Geometry check sheet. Reference: the model listing, model coordinates, mm. A direction names the side the tool comes from. Give positions to 0.01 mm unless a question says otherwise; leave off trailing zeros. Write each loop counter-clockwise with the first axis right and the second up, starting at its lowest first coordinate (ties: lowest second). Pieces come first, ordered by that corner, then holes. Notation, with made-up numbers: M -15,1 L 41,1 A32 cw 41,30 Z; hole C -8,-9 d5. An arc over 180 degrees is marked long. Write each question's results on one line, items separated by ' | '.
```python
from build123d import *

# Parameters (mm, degrees)
ESBO_O1_W       = 24.65
ESBO_O1_H       = 16
ESBO_O2_W       = 30
ESBO_O2_H       = 12
EXTRUS_O1_DEPTH = 25.1
CHANFRO1_SIZE   = 3
EXTRUS_O2_DEPTH = 1
ESBO_O5_W       = 8.5
ESBO_O5_H       = 6
EXTRUS_O3_DEPTH = 0.3
ESBO_O6_W       = 6.5
ESBO_O6_H       = 1
EXTRUS_O4_DEPTH = 10
ESBO_O7_R       = 2
EXTRUS_O5_DEPTH = 1
FILETE1_R       = 3
ESBO_O8_R       = 6
EXTRUS_O6_DEPTH = 2
ESBO_O9_R       = 3.5
EXTRUS_O7_DEPTH = 9.4
ESBO_O10_W      = 6.32455532
ESBO_O10_H      = 3.599019514
EXTRUS_O8_DEPTH = 6
ESBO_O11_W      = 30
ESBO_O11_H      = 9.10840564
EXTRUS_O9_DEPTH = 0.5
FILETE2_R       = 2


with BuildPart() as part:
    # Esboço1 → Revolução1 (revolve)
    with BuildSketch(Plane.XY, mode=Mode.PRIVATE) as revolu_o1_sk:
        with Locations((-12.325, 8)):
            Rectangle(ESBO_O1_W, ESBO_O1_H)
    revolve(revolu_o1_sk.sketch.rotate(Axis((0, 0, 0), (0, 1, 0)), 270), axis=Axis((0, 0, 0), (0, 1, 0)))

    # Esboço2 → Extrusão1 (add)
    with BuildSketch(Plane.XY):
        with Locations((0, 10)):
            Rectangle(ESBO_O2_W, ESBO_O2_H)
    extrude(amount=EXTRUS_O1_DEPTH)

    # Chanfro1
    chanfro1_edges = [part.edges().sort_by_distance(p)[0] for p in [
        (-15, 10, 25.1),
        (15, 10, 25.1),
    ]]
    chamfer(chanfro1_edges, length=CHANFRO1_SIZE)

    # Esboço4 → Extrusão2 (add)
    with BuildSketch(Plane.XY.offset(25.1)):
        Polygon((-12, 5), (-0.5, 5), (-0.5, 16), (0.5, 16), (0.5, 5), (12, 5), (12, 4), (-12, 4), align=None)
    extrude(amount=EXTRUS_O2_DEPTH)

    # Esboço5 → Extrusão3 (add)
    with BuildSketch(Plane.XY.offset(25.1)):
        with Locations((-7.75, 8)):
            Rectangle(ESBO_O5_W, ESBO_O5_H)
        with Locations((7.75, 8)):
            Rectangle(ESBO_O5_W, ESBO_O5_H)
    extrude(amount=EXTRUS_O3_DEPTH)

    # Esboço6 → Extrusão4 (add)
    with BuildSketch(Plane.XY.offset(25.4)):
        with Locations((-7.75, 8.5)):
            Rectangle(ESBO_O6_W, ESBO_O6_H)
        with Locations((7.75, 8.5)):
            Rectangle(ESBO_O6_W, ESBO_O6_H)
    extrude(amount=EXTRUS_O4_DEPTH)

    # Esboço7 → Extrusão5 (add)
    # profile 1 of 2: a face of its own
    with BuildSketch(Plane(origin=(0, 16, 0), x_dir=(1, 0, 0), z_dir=(0, 1, 0))):
        with BuildLine():
            ThreePointArc((-19.930990459, -14.504417235), (-23.303909287, -8.034320875), (-24.634983886, -0.860272594))
            Line((-24.634983886, -0.860272594), (-32, -1.117464624))
            Line((-32, -1.117464624), (-29.875626197, -14.851691567))
            Line((-29.875626197, -14.851691567), (-19.930990459, -14.504417235))
        make_face()
        with Locations(Location((-27.5, -11.35, 0), (0, 0, 270))):
            Circle(ESBO_O7_R, mode=Mode.SUBTRACT)
        with Locations(Location((-28.5, -4.35, 0), (0, 0, 270))):
            Circle(ESBO_O7_R, mode=Mode.SUBTRACT)
    # profile 2 of 2: a face of its own
    with BuildSketch(Plane(origin=(0, 16, 0), x_dir=(1, 0, 0), z_dir=(0, 1, 0))):
        with BuildLine():
            Line((32, -1.117464624), (24.634983886, -0.860272594))
            ThreePointArc((24.634983886, -0.860272594), (23.303909287, -8.034320875), (19.930990459, -14.504417235))
            Line((19.930990459, -14.504417235), (29.875626197, -14.851691567))
            Line((29.875626197, -14.851691567), (32, -1.117464624))
        make_face()
        with Locations(Location((27.5, -11.35, 0), (0, 0, 270))):
            Circle(ESBO_O7_R, mode=Mode.SUBTRACT)
        with Locations(Location((28.5, -4.35, 0), (0, 0, 270))):
            Circle(ESBO_O7_R, mode=Mode.SUBTRACT)
    extrude(amount=-EXTRUS_O5_DEPTH)

    # Filete1
    filete1_edges = [part.edges().sort_by_distance(p)[0] for p in [
        (-32, 15.5, 1.117464624),
        (-29.875626197, 15.5, 14.851691567),
        (32, 15.5, 1.117464624),
        (29.875626197, 15.5, 14.851691567),
    ]]
    fillet(filete1_edges, radius=FILETE1_R)

    # Esboço8 → Extrusão6 (add)
    with BuildSketch(Plane(origin=(0, 16, 0), x_dir=(1, 0, 0), z_dir=(0, 1, 0))):
        with Locations(Location((0, 12.65, 0), (0, 0, 90))):
            Circle(ESBO_O8_R)
    extrude(amount=EXTRUS_O6_DEPTH)

    # Esboço9 → Extrusão7 (add)
    with BuildSketch(Plane(origin=(0, 18, 0), x_dir=(1, 0, 0), z_dir=(0, 1, 0))):
        with Locations(Location((0, 12.65, 0), (0, 0, 270))):
            Circle(ESBO_O9_R)
    extrude(amount=EXTRUS_O7_DEPTH)

    # Esboço10 → Extrusão8 (cut)
    with BuildSketch(Plane(origin=(0, 27.4, 0), x_dir=(1, 0, 0), z_dir=(0, 1, 0))):
        with Locations((0, 9.350490243)):
            Rectangle(ESBO_O10_W, ESBO_O10_H)
    extrude(amount=-EXTRUS_O8_DEPTH, mode=Mode.SUBTRACT)

    # Esboço11 → Extrusão9 (cut)
    with BuildSketch(Plane(origin=(0, 16, 0), x_dir=(1, 0, 0), z_dir=(0, 1, 0))):
        with Locations((0, -24.114941559)):
            Rectangle(ESBO_O11_W, ESBO_O11_H)
    extrude(amount=-EXTRUS_O9_DEPTH, mode=Mode.SUBTRACT)

    # Filete2
    filete2_edges = [part.edges().sort_by_distance(p)[0] for p in [
        (4.5, 8.5, 35.4),
        (11, 8.5, 35.4),
        (-11, 8.5, 35.4),
        (-4.5, 8.5, 35.4),
    ]]
    fillet(filete2_edges, radius=FILETE2_R)


solid = part.part
```
Q1. Section check C-C (z = 0). Enter the section's corners in (x, y).
Answer key:
outline: M -24.65,0 L 24.65,0 L 24.65,16 L -24.65,16 Z
Q2. Material ranges on probe 1 along X at (y, z) = (15.3, 4.35); probe 2 along X at (y, z) = (8.5, 30); probe 3 along X at (y, z) = (15.8, 11.35), recorded low to high. Write a range as [from, to].
Answer key:
probe 1: x = [-31.5, -30.5], [-26.5, 26.5], [30.5, 31.5] | probe 2: x = [-11, -4.5], [4.5, 11] | probe 3: x = [-30.42, -29.5], [-25.5, 25.5], [29.5, 30.42]
Q3. Section check B-B (y = 13.25). Enter the section's corners in (x, z).
Answer key:
outline: M -15,19.56 A24.65 ccw long 15,19.56 L 15,22.1 L 12,25.1 L 0.5,25.1 L 0.5,26.1 L -0.5,26.1 L -0.5,25.1 L -12,25.1 L -15,22.1 Z
Q4. Depth check by flat-ended pin: P1, Ø1, axis at x = 0.5, z = -10.5, coming from the +Y side; P2, Ø3, axis at y = 6.5, z = -1, coming from the +X side; P3, Ø3.5, axis at x = 3, z = -11, coming from the +Y side; P4, Ø9.5, axis at x = 28.5, z = 9.5, coming from the -Y side. Enter the tip coordinate at first touch or a pass-through.
Answer key:
P1: stops at y = 21.4 | P2: stops at x = 24.65 | P3: stops at y = 27.4 | P4: stops at y = 15
Q5. Section check D-D (y = 10). Enter the section's corners in (x, z), then the cut area to 3 significant figures.
Answer key:
outline: M -15,19.56 A24.65 ccw long 15,19.56 L 15,22.1 L 12,25.1 L 12,25.4 L 3.5,25.4 L 3.5,25.1 L 0.5,25.1 L 0.5,26.1 L -0.5,26.1 L -0.5,25.1 L -3.5,25.1 L -3.5,25.4 L -12,25.4 L -12,25.1 L -15,22.1 Z | area: 1,970 mm2
Q6. Section check A-A (z = 27). Enter the section's corners in (x, y).
Answer key:
outline: M -11,8 L -4.5,8 L -4.5,9 L -11,9 Z; M 4.5,8 L 11,8 L 11,9 L 4.5,9 Z
Q7. Release check for a two-part mould opening along Y. For faces 4 (the face through (-8, 9, 30)), 5 (the face through (-8, 7, 25.4)), 6 (the face through (-15, 10, 21)), 7 (the face through (0, 0, 0)) record: released by +Y, released by -Y, zero draft, split by the parting line, or undercut.
Answer key:
face 4: released by +Y | face 5: undercut | face 6: zero draft | face 7: released by -Y
Q8. Access from +Z, -Z, +X, -X, +Y, -Y to the whole of each face (thin tool, end or side, straight path). Record for faces 1 (the face through (2.3, 16.99, -18.19)), 2 (the face through (15, 10, 21)), 3 (the face through (0, 15.5, 22)).
Answer key:
face 1: +Y | face 2: +Z, +X, +Y, -Y | face 3: +Z, +X, -X, +Y
